Check sheet for the modelled part. Datum: model origin and axes. Units: mm. A direction names the side the tool comes from. Coordinates: 2 decimals unless noted, no trailing zeros. Loops run counter-clockwise (first coordinate to the right, second up) from the corner with the lowest first, then second, coordinate; pieces in that order, holes last. Notation, with made-up numbers: (4.5, 14) -> (60.5, 14) arc R33 cw to (60.5, 46) -> close; hole circle Ø10 at (75, -25). An arc over 180 degrees is marked (long way). Use one line per item in the form item = value.
from build123d import *

# Parameters (mm, degrees)
F1_W          = 2.6
F1_H          = 10
F1_R          = 1.5
F2_DEPTH      = 1.3
F2_DEPTH_BACK = 1.3
F4_DEPTH      = 2.6010001


with BuildPart() as f2:
    # F1 (on Top) → F2 (new body, two sides)
    with BuildSketch(Plane.XY) as f2_sk:
        with BuildLine():
            Line((26.8950708133, -115.2), (0, -115.2))
            Line((0, -115.2), (0, -150.2))
            Line((0, -150.2), (11.25, -150.2))
            Line((11.25, -150.2), (11.25, -155.2))
            Line((11.25, -155.2), (23.3302194863, -155.2))
            Line((23.3302194863, -155.2), (28.3302194863, -155.2))
            add(Edge.make_bspline(
                [(28.3302194863, -155.2), (27.4209763541, -143.1676427283), (26.763234957, -130.0249441378), (26.8860792155, -115.9692984983), (26.8950708133, -115.2)],
                knots=[0.0235919502, 0.0235919502, 0.0235919502, 0.0235919502, 0.1835372396, 0.1927653287, 0.1927653287, 0.1927653287, 0.1927653287], degree=3))
        make_face()
        with Locations((12.8, -133.2)):
            Rectangle(F1_W, F1_H, mode=Mode.SUBTRACT)
        with BuildLine():
            ThreePointArc((24.8302194863, -145.2), (24.3908796581, -146.2606601718), (23.3302194863, -146.7))
            ThreePointArc((23.3302194863, -146.7), (21.8302194863, -145.2), (23.3302194863, -143.7))
            ThreePointArc((23.3302194863, -143.7), (24.3908796581, -144.1393398282), (24.8302194863, -145.2))
        make_face(mode=Mode.SUBTRACT)
        with BuildLine():
            ThreePointArc((24.8302194863, -120.2), (24.3908796581, -121.2606601718), (23.3302194863, -121.7))
            ThreePointArc((23.3302194863, -121.7), (22.2695593146, -119.1393398282), (24.8302194863, -120.2))
        make_face(mode=Mode.SUBTRACT)
        with BuildLine():
            add(Edge.make_bspline(
                [(-28.3302194863, -155.2), (-27.4209763541, -143.1676427283), (-26.763234957, -130.0249441378), (-26.8860792155, -115.9692984983), (-26.8950708133, -115.2)],
                knots=[0.0235919502, 0.0235919502, 0.0235919502, 0.0235919502, 0.1835372396, 0.1927653287, 0.1927653287, 0.1927653287, 0.1927653287], degree=3))
            Line((-28.3302194863, -155.2), (-11.25, -155.2))
            Line((-11.25, -155.2), (-11.25, -150.2))
            Line((-11.25, -150.2), (0, -150.2))
            Line((0, -150.2), (0, -115.2))
            Line((0, -115.2), (-26.8950708133, -115.2))
        make_face()
        with Locations((-23.3302194863, -145.2)):
            Circle(F1_R, mode=Mode.SUBTRACT)
        with Locations((-23.3302194863, -120.2)):
            Circle(F1_R, mode=Mode.SUBTRACT)
        with Locations((-12.8, -133.2)):
            Rectangle(F1_W, F1_H, mode=Mode.SUBTRACT)
    extrude(amount=F2_DEPTH)
    extrude(f2_sk.sketch, amount=-F2_DEPTH_BACK)

    # F3 (on face) → F4 (cut, through all)
    with BuildSketch(Plane.XY.offset(1.3)):
        Polygon((35.375, 8.25), (27.6897869255, 8.25), (27.6897869255, -6.25), (35.375, -6.25), (39.6897869255, -6.25), (39.6897869255, 8.25), align=None)
        Polygon((-27.6897869255, -6.25), (-27.6897869255, 8.25), (-35.375, 8.25), (-39.6897869255, 8.25), (-39.6897869255, -6.25), (-35.375, -6.25), align=None)
    extrude(amount=-F4_DEPTH, mode=Mode.SUBTRACT)


solid = f2.part
(1) Tool access check on faces 1 (the flat face through (20, -155.2, 0)), 2 (the flat face through (13, -128.2, 0)), 3 (the flat face through (-11.25, -153, 0)). Record the directions out of +Z, -Z, +X, -X, +Y, -Y that give a thin tool (end or side, any length) a straight path to the whole face; none if there is none.
Established:
face_1 = +Z, -Z, +X, -X, -Y
face_2 = +Z, -Z
face_3 = +Z, -Z, -Y
(2) Section check A-A, the plane x = -8.5. Record the boundary of the cut face in (y, z), plus the area to 3 significant figures.
Established:
outline = (-150.2, -1.3) -> (-115.2, -1.3) -> (-115.2, 1.3) -> (-150.2, 1.3) -> close
area = 91.0 mm²
(3) Go/stop test with flat-tipped pins: P1, Ø1.4, axis at y = -131, z = 0.5, coming from the +X side; P2, Ø5, axis at x = -23.33, y = -120.2, coming from the -Z side; P3, Ø1.3, axis at x = 5.5, z = 0, coming from the -Y side; P4, Ø1.4, axis at y = -131.5, z = -0.5, coming from the -X side. Record where each tip stops, or that it passes through.
Established:
P1 = 27.05
P2 = -1.3
P3 = -150.2
P4 = -27.07
(4) Section check B-B, the plane z = -0.6. Give the number of separate pieces and of enclosed holes in the cut face, plus the area to 3 significant figures.
Established:
separate_pieces = 1
enclosed_holes = 6
area = 1,990 mm²
(5) Mould release check, pull along Y, two halves, no side actions. Record for faces 4 (the flat face through (0, -135, -1.3)), 5 (the cylindrical face through (-23.525, -118.713, -0.018)), 6 (the flat face through (13, -138.2, 0)), 7 (the flat face through (0, -115.2, 0)): +Y half, -Y half, draft (parallel to the pull), parting line (faces both ways), or undercut.
Established:
face_4 = draft
face_5 = undercut
face_6 = undercut
face_7 = +Y half
(6) Scan lines: line 1 along X through (y, z) = (-120.2, 0.55); line 2 along Y through (x, z) = (-24.5, 0.25); line 3 along X through (y, z) = (-132.5, 0.6). Record each from-to range of solid material in increasing order.
Established:
line_1 = -26.87 to -24.83, -21.83 to 21.83, 24.83 to 26.87
line_2 = -155.2 to -146.14, -144.26 to -121.14, -119.26 to -115.2
line_3 = -27.08 to -14.1, -11.5 to 11.5, 14.1 to 27.08
